```python
from build123d import *

# Parameters (mm, degrees)
SKETCH12_W           = 90
SKETCH12_H           = 126.33
BOSS_EXTRUDE10_DEPTH = 12.7
SKETCH15_R           = 25.4
BOSS_EXTRUDE11_DEPTH = 15
SKETCH23_R           = 22.5
CUT_EXTRUDE7_DEPTH   = 200.671813095
FILLET2_R            = 12.8
SKETCH25_W           = 29.125
SKETCH25_H           = 12.7
CUT_EXTRUDE9_DEPTH   = 199.309210439
CUT_EXTRUDE10_DEPTH  = 199.309210439
CHAMFER1_SIZE        = 1


with BuildPart() as part:
    # Sketch12 → Boss-Extrude10 (new body)
    with BuildSketch(Plane.XY):
        with Locations((107.125849364, 63.165)):
            Rectangle(SKETCH12_W, SKETCH12_H)
    extrude(amount=BOSS_EXTRUDE10_DEPTH)

    # Sketch15 → Boss-Extrude11 (add)
    with BuildSketch(Plane.XY.offset(12.7)):
        with Locations(Location((107.125849364, 38.627603634, 0), (0, 0, 180))):
            Circle(SKETCH15_R)
    extrude(amount=BOSS_EXTRUDE11_DEPTH)

    # Sketch23 → Cut-Extrude7 (cut, through all)
    with BuildSketch(Plane.XY.offset(27.7)):
        with Locations((107.125849364, 38.627603634)):
            Circle(SKETCH23_R)
    extrude(amount=-CUT_EXTRUDE7_DEPTH, mode=Mode.SUBTRACT)

    # Fillet2
    fillet2_edges = [part.edges().sort_by_distance(p)[0] for p in [
        (62.125849364, 0, 6.35),
        (152.125849364, 0, 6.35),
    ]]
    fillet(fillet2_edges, radius=FILLET2_R)

    # Sketch25 → Cut-Extrude9 (cut, through all)
    with BuildSketch(Plane.XY.offset(12.7)):
        with Locations((76.688349364, 119.98)):
            Rectangle(SKETCH25_W, SKETCH25_H)
        with Locations((137.563349364, 119.98)):
            Rectangle(SKETCH25_W, SKETCH25_H)
    extrude(amount=-CUT_EXTRUDE9_DEPTH, mode=Mode.SUBTRACT)

    # Sketch27 → Cut-Extrude10 (cut, through all)
    with BuildSketch(Plane.XY.offset(12.7)):
        Polygon((147.917849364, 113.63), (147.917849364, 108.931), (150.279849364, 108.931), (150.279849364, 103.089), (147.917849364, 103.089), (147.917849364, 98.39), (141.313849364, 98.39), (141.313849364, 103.089), (138.951849364, 103.089), (138.951849364, 108.931), (141.313849364, 108.931), (141.313849364, 113.63), align=None)
        Polygon((72.937849364, 103.089), (75.299849364, 103.089), (75.299849364, 108.931), (72.937849364, 108.931), (72.937849364, 113.63), (66.333849364, 113.63), (66.333849364, 108.931), (63.971849364, 108.931), (63.971849364, 103.089), (66.333849364, 103.089), (66.333849364, 98.39), (72.937849364, 98.39), align=None)
    extrude(amount=-CUT_EXTRUDE10_DEPTH, mode=Mode.SUBTRACT)

    # Chamfer1
    chamfer1_edges = [part.edges().sort_by_distance(p)[0] for p in [
        (132.525849364, 38.627603634, 27.7),
    ]]
    chamfer(chamfer1_edges, length=CHAMFER1_SIZE)


solid = part.part
```
The listing builds one solid part. Answer for the finished solid, in the listing's coordinates (mm). A direction names the side the tool comes from. Give positions to 0.01 mm unless a question says otherwise; leave off trailing zeros. Order: outer loops, then holes, each group sorted by start corner. A loop starts at its lowest first (then second) coordinate and runs counter-clockwise, first axis right, second up. Notation, with made-up numbers: (1.5, 63) - (14.5, 63) arc R26 cw to (14.5, 96) - close; hole circle Ø9 at (64, -2.5). An arc over 180 degrees is marked (long way). Answer in a Markdown table with one row per item. Add a question column.
Q1. For a pull along X with two mould halves and no side action, classify faces 5 (the flat face through (107, 126.33, 6)), 6 (the flat face through (123.001, 120, 6)), 7 (the flat face through (66.334, 101, 6)) as released by +X, released by -X, zero draft, split by the parting line, or undercut.
Q2. The part is cut by section C-C (z = 20). Determine the outline of the cut face in (x, y), then the cut area to 3 significant figures.
Q3. The part is cut by section B-B (y = 81). Determine the outline of the cut face in (x, z), then the cut area to 3 significant figures.
Q4. The part is cut by section A-A (x = 77). Determine the outline of the cut face in (y, z), then the cut area to 3 significant figures.
Q5. Find the intervals of material crossed by line 1 along X through (y, z) = (106.5, 1.75); line 2 along Z through (x, y) = (128.5, 78.5); line 3 along Y through (x, z) = (131, 7.25), in increasing order. Write a range as [from, to].
Q6. Which of the six approach directions +Z, -Z, +X, -X, +Y, -Y give full straight-line access (tool end or side, diameter ignored) to faces 1 (the flat face through (63.972, 106, 6)), 2 (the cylindrical face through (127.282, 54.083, 19.602)), 3 (the flat face through (82, 113.63, 6)), 4 (the flat face through (145, 98.39, 6))?
Q7. Given P1, Ø1.3, axis at x = 149.5, z = 3, coming from the +Y side; P2, Ø4, axis at y = 117.5, z = 8.5, coming from the +X side; P3, Ø14, axis at y = 123, z = 3, coming from the -X side, each flat-ended and moving along its own axis, determine where each tip first touches the part or whether it passes through.
Determined:
| question | item | result |
|---|---|---|
| 1 | face 5 | zero draft |
| 1 | face 6 | released by +X |
| 1 | face 7 | undercut |
| 2 | outline | circle Ø50.8 at (107.13, 38.63); hole circle Ø45 at (107.13, 38.63) |
| 2 | area | 436 mm² |
| 3 | outline | (62.13, 0) - (152.13, 0) - (152.13, 12.7) - (62.13, 12.7) - close |
| 3 | area | 1,140 mm² |
| 4 | outline | (0, 0) - (113.63, 0) - (113.63, 12.7) - (0, 12.7) - close |
| 4 | area | 1,440 mm² |
| 5 | line 1 | x = [62.13, 63.97], [75.3, 138.95], [150.28, 152.13] |
| 5 | line 2 | z = [0, 12.7] |
| 5 | line 3 | y = [0, 113.63] |
| 6 | face 1 | +Z, -Z |
| 6 | face 2 | +Z |
| 6 | face 3 | +Z, -Z, -X, +Y |
| 6 | face 4 | +Z, -Z, +Y |
| 7 | P1 | stops at y = 113.63 |
| 7 | P2 | stops at x = 123 |
| 7 | P3 | stops at x = 91.25 |
